For this review, use the dimensioned drawing (mm, ordinates from the lowest corner) and the shaded views. Round coordinates to 2 decimals unless told otherwise and drop trailing zeros. Write each loop counter-clockwise with the first axis right and the second up, starting at its lowest first coordinate (ties: lowest second). Pieces come first, ordered by that corner, then holes.
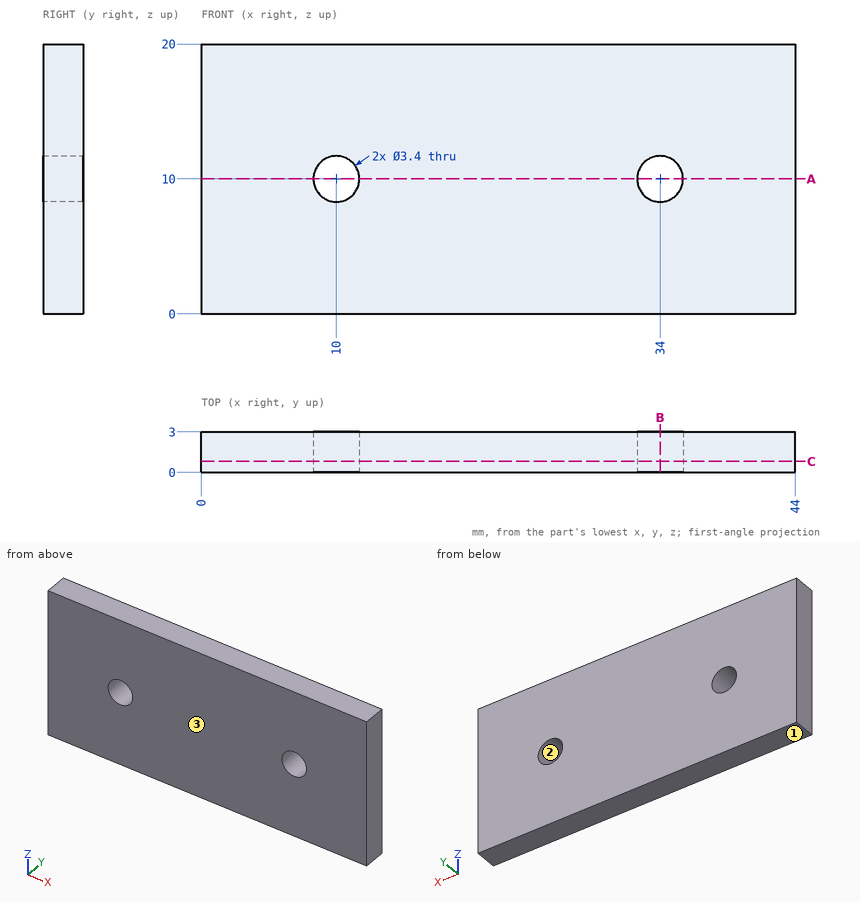
(1) We need section C-C, the plane y = 0.8. Give the boundary of the cut face in (x, z), and give its area (3 significant figures).
Geometry check:
outline: (0, 0) - (44, 0) - (44, 20) - (0, 20) - close; hole circle Ø3.4 at (10, 10); hole circle Ø3.4 at (34, 10)
area: 862 mm2
(2) Mouldability with a two-part tool opening along Z and no side actions: class the marked faces 1, 2 and 3 as pulls with the +Z half, pulls with the -Z half, needs draft (parallel to the pull), parting line crosses it, or undercut.
Geometry check:
face 1: pulls with the -Z half
face 2: undercut
face 3: needs draft
(3) For line 1 along X through (y, z) = (0.8, 10); line 2 along Z through (x, y) = (10, 1.7); line 3 along X through (y, z) = (2.5, 9), list the stretches that pass through material, from the lowest coordinate up.
Geometry check:
line 1: x = 0 to 8.3, 11.7 to 32.3, 35.7 to 44
line 2: z = 0 to 8.3, 11.7 to 20
line 3: x = 0 to 8.63, 11.37 to 32.63, 35.37 to 44
(4) For pin 1 Ø4.5 at (x, z) = (34, 10) entering from -Y, flat-tipped, find the tip position at first contact; note if it passes through.
Geometry check:
pin 1: stops at y = 0
(5) We need section B-B, the plane x = 34. Give the boundary of the cut face in (y, z).
Geometry check:
outline: (0, 0) - (3, 0) - (3, 8.3) - (0, 8.3) - close; (0, 11.7) - (3, 11.7) - (3, 20) - (0, 20) - close
(6) We need section A-A, the plane z = 10. Give the boundary of the cut face in (x, y).
Geometry check:
outline: (0, 0) - (8.3, 0) - (8.3, 3) - (0, 3) - close; (11.7, 0) - (32.3, 0) - (32.3, 3) - (11.7, 3) - close; (35.7, 0) - (44, 0) - (44, 3) - (35.7, 3) - close
